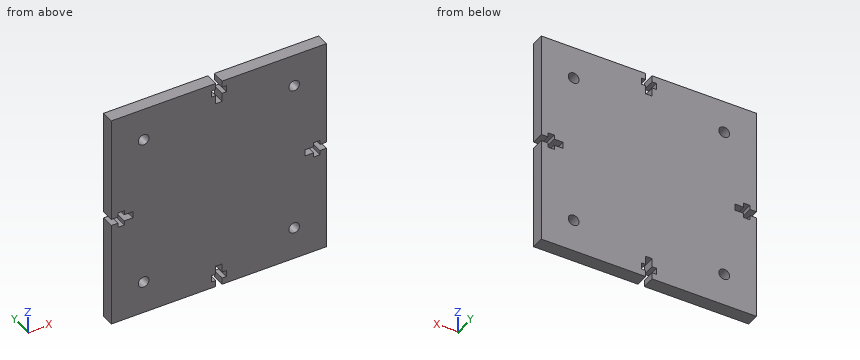
from build123d import *

# Parameters (mm, degrees)
SKETCH1_W           = 100
SKETCH1_H           = 100
BOSS_EXTRUDE1_DEPTH = 6
CUT_EXTRUDE1_DEPTH  = 7
SKETCH4_R           = 2.5
CUT_EXTRUDE3_DEPTH  = 7
CUT_EXTRUDE4_DEPTH  = 10


with BuildPart() as part:
    # Sketch1 → Boss-Extrude1 (new body)
    with BuildSketch(Plane(origin=(0, 0, 0), x_dir=(1, 0, 0), z_dir=(0, 1, 0))):
        with Locations((50, -50)):
            Rectangle(SKETCH1_W, SKETCH1_H)
    extrude(amount=BOSS_EXTRUDE1_DEPTH)

    # Sketch2 → Cut-Extrude1 (cut, through all)
    with BuildSketch(Plane(origin=(0, 6, 0), x_dir=(1, 0, 0), z_dir=(0, 1, 0))):
        Polygon((48.5, 0), (51.5, 0), (51.5, -3), (53.5, -3), (53.5, -6), (51.5, -6), (51.5, -10), (48.5, -10), (48.5, -6), (46.5, -6), (46.5, -3), (48.5, -3), align=None)
        Polygon((48.5, -100), (48.5, -97), (46.5, -97), (46.5, -94), (48.5, -94), (48.5, -90), (51.5, -90), (51.5, -94), (53.5, -94), (53.5, -97), (51.5, -97), (51.5, -100), align=None)
    extrude(amount=-CUT_EXTRUDE1_DEPTH, mode=Mode.SUBTRACT)

    # Sketch4 → Cut-Extrude3 (cut, through all)
    with BuildSketch(Plane(origin=(0, 0, 0), x_dir=(-1, 0, 0), z_dir=(0, -1, 0))):
        with Locations((-15, -85)):
            Circle(SKETCH4_R)
        with Locations((-85, -85)):
            Circle(SKETCH4_R)
        with Locations((-85, -15)):
            Circle(SKETCH4_R)
        with Locations((-15, -15)):
            Circle(SKETCH4_R)
    extrude(amount=-CUT_EXTRUDE3_DEPTH, mode=Mode.SUBTRACT)

    # Sketch5 → Cut-Extrude4 (cut)
    with BuildSketch(Plane.XZ):
        Polygon((0, 51.193613504), (0, 50), (0, 48.5), (3, 48.5), (3, 46.439353032), (6, 46.439353032), (6, 48.5), (10, 48.5), (10, 50), (10, 51.5), (6, 51.5), (6, 53.5), (3, 53.5), (3, 51.5), (0, 51.5), align=None)
        Polygon((100, 48.5), (100, 50), (100, 51.5), (97, 51.5), (97, 53.5), (94, 53.5), (94, 51.5), (90, 51.5), (90, 50), (90, 48.5), (94, 48.5), (94, 46.439353032), (97, 46.439353032), (97, 48.5), align=None)
    extrude(amount=-CUT_EXTRUDE4_DEPTH, mode=Mode.SUBTRACT)


solid = part.part
Can you work these out from the model? Positions are in its coordinate system, mm. Round coordinates to 2 decimals unless told otherwise and drop trailing zeros. Loops run counter-clockwise (first coordinate to the right, second up) from the corner with the lowest first, then second, coordinate; pieces in that order, holes last. Notation, with made-up numbers: (-9.5, -5) - (32.5, -5) arc R26 ccw to (32.5, 28) - close; hole circle Ø1 at (44.5, 54). An arc over 180 degrees is marked (long way). Write item = value, one per line. Start each with the question number.
(1) If I drill on probe 1 along Z at (x, y) = (85, 4.4); probe 2 along Z at (x, y) = (47.5, 0.7), over which ranges is the centre line in solid material (lowest first)? Write a range as [from, to].
(2) For P1, Ø0.6, axis at y = 2, z = 53, coming from the -X side, with a flat end and sliding along its axis, tell me the tip position at first contact or that it passes through.
(3) If we section it at A-A (z = 15): Please give me the cut outline in (x, y), and give its area (3 significant figures).
(4) If we section it at B-B (x = 15): Please give me the cut outline in (y, z).
(5) If we section it at C-C (y = 2.2): Give the number of separate pieces and of enclosed holes in the cut face, and give its area (3 significant figures).
(6) If we section it at D-D (z = 50): Please give me the cut outline in (x, y), and give its area (3 significant figures).
Ans:
q1.probe_1 = [0, 12.5], [17.5, 82.5], [87.5, 100]
q1.probe_2 = [0, 3], [6, 94], [97, 100]
q2.P1 = 0
q3.outline = (0, 0) - (12.5, 0) - (12.5, 6) - (0, 6) - close; (17.5, 0) - (82.5, 0) - (82.5, 6) - (17.5, 6) - close; (87.5, 0) - (100, 0) - (100, 6) - (87.5, 6) - close
q3.area = 540 mm²
q4.outline = (0, 0) - (6, 0) - (6, 12.5) - (0, 12.5) - close; (0, 17.5) - (6, 17.5) - (6, 82.5) - (0, 82.5) - close; (0, 87.5) - (6, 87.5) - (6, 100) - (0, 100) - close
q5.separate_pieces = 1
q5.enclosed_holes = 4
q5.area = 9,750 mm²
q6.outline = (10, 0) - (90, 0) - (90, 6) - (10, 6) - close
q6.area = 480 mm²
